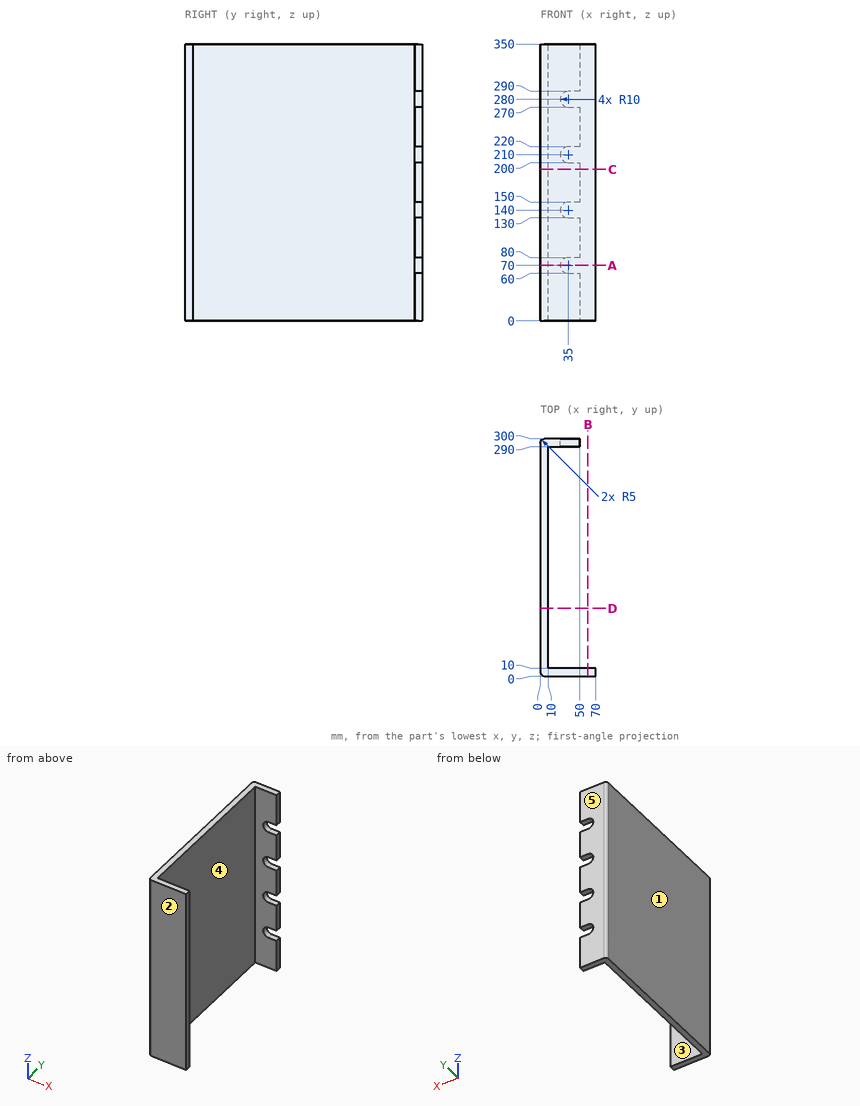
Geometry: see drawing. Coordinates: mm, zero at the bounding-box minimum. A direction names the side the tool comes from. Coordinates: 2 decimals unless noted, no trailing zeros. Loops run counter-clockwise (first coordinate to the right, second up) from the corner with the lowest first, then second, coordinate; pieces in that order, holes last. Notation, with made-up numbers: M 61,-5.75 L 72,-5.75 A15 ccw 72,18.25 Z; hole C 16,8 d1. An arc over 180 degrees is marked long. Answer in a Markdown table with one row per item.
1. Draft query along Y for the marked faces 1, 2 and 3. Return one class per face: pulls with the +Y half, pulls with the -Y half, needs draft (parallel to the pull), parting line crosses it, or undercut.
Response:
| item | result |
|---|---|
| face 1 | needs draft |
| face 2 | pulls with the -Y half |
| face 3 | undercut |
2. Section A-A, the plane z = 70. Output: boundary loops of the cut face in (x, y).
Response:
| item | result |
|---|---|
| outline | M 0,5 A5 ccw 5,0 L 70,0 L 70,10 L 10,10 L 10,290 L 25,290 L 25,300 L 5,300 A5 ccw 0,295 Z |
3. First-contact query: pin 1 (11 mm diameter, centred on y = 294, z = 237.5, fed in from +X); pin 2 (2 mm diameter, centred on x = 54, z = 201, fed in from +Y). Flat tips, straight axial feed; report the tip coordinate or a pass-through.
Response:
| item | result |
|---|---|
| pin 1 | stops at x = 50 |
| pin 2 | stops at y = 10 |
4. Material intervals for line 1 (Y direction, x = 11, z = 32.5); line 2 (X direction, y = 226, z = 265.5), sorted ascending.
Response:
| item | result |
|---|---|
| line 1 | y = 0 to 10, 290 to 300 |
| line 2 | x = 0 to 10 |
5. Reachability of the marked faces 4 and 5 from +Z, -Z, +X, -X, +Y, -Y: full face, straight path, thin tool, end or side. Return the list, or none.
Response:
| item | result |
|---|---|
| face 4 | +Z, -Z, +X |
| face 5 | +Z, -Z, +X, -X, +Y |
6. Section C-C, the plane z = 191.5. Output: boundary loops of the cut face in (x, y), then the cut area to 3 significant figures.
Response:
| item | result |
|---|---|
| outline | M 0,5 A5 ccw 5,0 L 70,0 L 70,10 L 10,10 L 10,290 L 50,290 L 50,300 L 5,300 A5 ccw 0,295 Z |
| area | 3,990 mm2 |
7. Section B-B, the plane x = 60. Output: boundary loops of the cut face in (y, z).
Response:
| item | result |
|---|---|
| outline | M 0,0 L 10,0 L 10,350 L 0,350 Z |
